Geometry: final body of the model. Coordinates: model frame, mm. A direction names the side the tool comes from. Give positions to 0.01 mm unless a question says otherwise; leave off trailing zeros. Write each loop counter-clockwise with the first axis right and the second up, starting at its lowest first coordinate (ties: lowest second). Pieces come first, ordered by that corner, then holes. Notation, with made-up numbers: (20.25, 51) - (68.25, 51) arc R35 cw to (68.25, 85) - close; hole circle Ø4 at (39, -38.75). An arc over 180 degrees is marked (long way). Use CSV: the item, a comma, the result in double quotes. Start each with the question number.
(1) Section A-A on z = 0.7. Count the separate pieces of the cut face and the enclosed holes in it, and give its area (3 significant figures).
(2) Section B-B on y = 10. Output: boundary loops of the cut face in (x, z).
(3) Line query: probe 1 along Y at (x, z) = (11, 1.35); probe 2 along Y at (x, z) = (5.75, 2.8); probe 3 along Y at (x, z) = (8.25, 1.35). Output: solid intervals per line, ascending. Write a range as [from, to].
(4) Section C-C on y = 34. Output: boundary loops of the cut face in (x, z), and give its area (3 significant figures).
(5) Draft query along X for faces 1 (the cylindrical face through (0.285, 0.301, 1.521)), 2 (the cylindrical face through (3.037, 3.45, 1.479)), 3 (the flat face through (7, 0, 1)). Return one class per face: released by +X, released by -X, zero draft, split by the parting line, or undercut.
(6) Section D-D on y = 15. Output: boundary loops of the cut face in (x, z), and give its area (3 significant figures).
(7) Reachability of faces 4 (the cylindrical face through (11.674, 7.226, 1.479)), 5 (the flat face through (0, 18, 1)) from +Z, -Z, +X, -X, +Y, -Y: full face, straight path, thin tool, end or side. Return the list, or none.
(8) First-contact query: pin 1 Ø1 at (x, y) = (4.5, 25) entering from -Z. Flat tip, straight axial feed; report the tip coordinate or a pass-through.
from build123d import *

# Parameters (mm, degrees)
SKETCH_1_W          = 15
SKETCH_1_H          = 37
SKETCH_1_R          = 1.45
EXTRUDE_1_DEPTH     = 3
CUT_EXTRUDE_1_DEPTH = 10
FILLET_3_R          = 1


with BuildPart() as part:
    # 草图1 → 凸台-拉伸1 (new body)
    with BuildSketch(Plane.XY):
        with Locations((7.5, 18.5)):
            Rectangle(SKETCH_1_W, SKETCH_1_H)
        with Locations((4, 18.5)):
            Circle(SKETCH_1_R, mode=Mode.SUBTRACT)
        with Locations((11, 18.5)):
            Circle(SKETCH_1_R, mode=Mode.SUBTRACT)
    extrude(amount=EXTRUDE_1_DEPTH)

    # 草图2 → 切除-拉伸1 (cut)
    with BuildSketch(Plane.XY.offset(3)):
        Polygon((1.434880502, 34.882599316), (12.379202278, 34.543765824), (12.379202278, 24.936066313), align=None)
        Polygon((2.790214468, 30.545530624), (2.790214468, 22.074693336), (13.056869261, 22.074693336), align=None)
        Polygon((4.857098766, 15.365790203), (12.379202278, 15.365790203), (12.379202278, 5.133018759), align=None)
        Polygon((2.790214468, 14.450939776), (2.790214468, 3.215813333), (12.379202278, 2.117400684), align=None)
    extrude(amount=-CUT_EXTRUDE_1_DEPTH, mode=Mode.SUBTRACT)

    # 圆角3
    fillet_3_edges = [part.edges().sort_by_distance(p)[0] for p in [
        (2.790214468, 30.545530624, 1.5),
        (13.056869261, 22.074693336, 1.5),
        (2.790214468, 22.074693336, 1.5),
        (12.379202278, 5.133018759, 1.5),
        (4.857098766, 15.365790203, 1.5),
        (12.379202278, 15.365790203, 1.5),
        (2.790214468, 14.450939776, 1.5),
        (12.379202278, 2.117400684, 1.5),
        (2.790214468, 3.215813333, 1.5),
        (12.379202278, 24.936066313, 1.5),
        (1.434880502, 34.882599316, 1.5),
        (12.379202278, 34.543765824, 1.5),
        (0, 37, 1.5),
        (15, 37, 1.5),
        (15, 0, 1.5),
        (0, 0, 1.5),
    ]]
    fillet(fillet_3_edges, radius=FILLET_3_R)


solid = part.part
Check values:
1,separate pieces,"1"
1,enclosed holes,"6"
1,area,"364 mm²"
2,outline,"(0, 0) - (2.79, 0) - (2.79, 3) - (0, 3) - close; (6.25, 0) - (8.8, 0) - (8.8, 3) - (6.25, 3) - close; (12.38, 0) - (15, 0) - (15, 3) - (12.38, 3) - close"
3,probe 1,"y = [0, 2.89], [3.87, 7.26], [15.37, 17.05], [19.95, 22.39], [23.76, 26.27], [34.59, 37]"
3,probe 2,"y = [0, 2.88], [10.64, 22.07], [28.1, 30.96], [34.75, 37]"
3,probe 3,"y = [0, 2.59], [7.43, 10.75], [15.37, 22.07], [26.04, 28.69], [34.67, 37]"
4,outline,"(0, 0) - (3.13, 0) - (3.13, 3) - (0, 3) - close; (12.28, 0) - (15, 0) - (15, 3) - (12.28, 3) - close"
4,area,"17.6 mm²"
5,face 1,"released by -X"
5,face 2,"undercut"
5,face 3,"zero draft"
6,outline,"(0, 0) - (6.06, 0) - (6.06, 3) - (0, 3) - close; (12.15, 0) - (15, 0) - (15, 3) - (12.15, 3) - close"
6,area,"26.7 mm²"
7,face 4,"+Z, -Z"
7,face 5,"+Z, -Z, -X, +Y, -Y"
8,pin 1,"passes through"
